The model under review builds one solid part; all positions refer to its coordinate system, in mm. Round coordinates to 2 decimals unless told otherwise and drop trailing zeros. Order: outer loops, then holes, each group sorted by start corner. A loop starts at its lowest first (then second) coordinate and runs counter-clockwise, first axis right, second up. Notation, with made-up numbers: (0, 10) -> (31, 10) arc R19 cw to (31, 37) -> close; hole circle Ø2 at (79, 71). An arc over 180 degrees is marked (long way). Return JSON: item names as keys, results as strings. Group by question number.
from build123d import *

# Parameters (mm, degrees)
SKETCH_W        = 220
SKETCH_H        = 220
PAD_DEPTH       = 3
SKETCH001_R     = 3.2
POCKET_DEPTH    = 3.001
SKETCH002_R     = 2.75
POCKET001_DEPTH = 5
FILLET_R        = 5.5


with BuildPart() as part:
    # Sketch → Pad (new body)
    with BuildSketch(Plane.XY):
        Rectangle(SKETCH_W, SKETCH_H)
    extrude(amount=PAD_DEPTH)

    # Sketch001 (on Face6 of Pad) → Pocket (cut, through all)
    with BuildSketch(Plane.XY.offset(3)):
        with Locations((-104.5, 104.5)):
            Circle(SKETCH001_R)
        with Locations((104.5, 104.5)):
            Circle(SKETCH001_R)
        with Locations((104.5, -104.5)):
            Circle(SKETCH001_R)
        with Locations((-104.5, -104.5)):
            Circle(SKETCH001_R)
    extrude(amount=-POCKET_DEPTH, mode=Mode.SUBTRACT)

    # Sketch002 (on Face5 of Pocket) → Pocket001 (cut)
    with BuildSketch(Plane.XY.offset(3)):
        with Locations((-80, 80)):
            Circle(SKETCH002_R)
        with Locations((80, 80)):
            Circle(SKETCH002_R)
        with Locations((-80, -80)):
            Circle(SKETCH002_R)
        with Locations((80, -80)):
            Circle(SKETCH002_R)
    extrude(amount=-POCKET001_DEPTH, mode=Mode.SUBTRACT)

    # Fillet
    fillet_edges = [part.edges().sort_by_distance(p)[0] for p in [
        (-110, -110, 1.5),
        (110, -110, 1.5),
        (110, 110, 1.5),
        (-110, 110, 1.5),
    ]]
    fillet(fillet_edges, radius=FILLET_R)


solid = part.part
Item 1: Consider section A-A on x = 80. State the section outline as (y, z) points, plus the area to 3 significant figures.
Item 2: The part is to be moulded in two halves that separate along X. For faces 1 (the face through (-2, 2, 0)), 2 (the face through (-108.43, -108.35, 1.52)), 3 (the face through (-82.747, -79.879, 1.521)), say which applies: +X half, -X half, draft (parallel to the pull), parting line (faces both ways), or undercut.
Item 3: Insertion check: pin 1 Ø4 at (x, y) = (104.5, -104.5) entering from -Z. The pin has a flat end and moves straight along its axis. Give the tip position at first contact, or say it passes through.
Item 4: Wall thickness on line 1 along Y through (x, z) = (-104.5, 1.3); line 2 along Y through (x, z) = (-80, 1.8): over which ranges is each line inside the solid? List them lowest first.
Values:
{
 "1": {"outline": "(-110, 0) -> (-82.75, 0) -> (-82.75, 3) -> (-110, 3) -> close; (-77.25, 0) -> (77.25, 0) -> (77.25, 3) -> (-77.25, 3) -> close; (82.75, 0) -> (110, 0) -> (110, 3) -> (82.75, 3) -> close", "area": "627 mm^2"},
 "2": {"face 1": "draft", "face 2": "-X half", "face 3": "undercut"},
 "3": {"pin 1": "through"},
 "4": {"line 1": "-110 to -107.7, -101.3 to 101.3, 107.7 to 110", "line 2": "-110 to -82.75, -77.25 to 77.25, 82.75 to 110"}
}
